Here's how the part is built. I have some questions about the finished solid (model axes, mm). Coordinates: 2 decimals unless noted, no trailing zeros. Write each loop counter-clockwise with the first axis right and the second up, starting at its lowest first coordinate (ties: lowest second). Pieces come first, ordered by that corner, then holes. Notation, with made-up numbers: (-33.75, -10.75) -> (-24.75, -10.75) arc R14 cw to (-24.75, 16.25) -> close; hole circle Ø3 at (27, 19.5). An arc over 180 degrees is marked (long way). Use a Markdown table: item, result. Add a question column.
Item 1: Imagine slicing it at C-C, the plane z = 182. Write out the boundary of the cut face in (x, y), and give its area (3 significant figures).
Item 2: If I drill on line 1 along Y through (x, z) = (0.75, 92); line 2 along X through (y, z) = (6, 53); line 3 along Y through (x, z) = (1.5, 62), over which ranges is the centre line in solid material (lowest first)? Write a range as from..to.
Item 3: Will these pins go through, and if not, where does the flat tip stop? pin 1 Ø6 at (x, y) = (-3, 0.5) entering from -Z; pin 2 Ø2 at (x, z) = (7.5, 135.5) entering from -Y; pin 3 Ø1.5 at (y, z) = (-7.5, 146) entering from +X; pin 4 Ø1.5 at (x, z) = (1, 33.5) entering from -Y.
Autodesk Inventor part; units mm, degrees
ref_plane "YZ Plane" through (0, 0, 0) normal (1, 0, 0) x (0, 1, 0)
ref_plane "XZ Plane" through (0, 0, 0) normal (0, 1, 0) x (-1, 0, 0)
ref_plane "XY Plane" through (0, 0, 0) normal (0, 0, 1) x (1, 0, 0)
sketch "Skizze1" plane through (0, 0, 0) normal (0, 0, 1) x (1, 0, 0)
  circle A0 centre (0, 0) radius 8
  circle A1 centre (0, 0) radius 10.05
  dimension "d0" = 20.1
  dimension "d1" = 2.05
extrude "Extrusion1" add sketch "Skizze1" along normal blind 286
sketch "Skizze2" plane through (0, 0, 286) normal (0, 0, 1) x (1, 0, 0)
  circle A0 centre (0, 0) radius 10.05
  circle A1 centre (0, 0) radius 9.75
  dimension "d4" = 19.5
extrude "Extrusion2" cut sketch "Skizze2" against normal through all
sketch "Skizze3" plane through (0, 0, 0) normal (0, 0, -1) x (-1, 0, 0)
  circle A0 centre (0, 0) radius 9.75
  circle A1 centre (0, 0) radius 8
  circle A2 centre (0, 0) radius 10
  dimension "d7" = 20
extrude "Extrusion3" add sketch "Skizze3" against normal blind 9 contours A2
sketch "Skizze4" plane through (0, 0, 286) normal (0, 0, 1) x (1, 0, 0)
  circle A0 centre (0, 0) radius 9.75
  circle A1 centre (0, 0) radius 8
  circle A2 centre (0, 0) radius 9
  dimension "d10" = 18
extrude "Extrusion4" cut sketch "Skizze4" against normal blind 50 contours A0
sketch "Skizze5" plane through (0, 0, 0) normal (0, 1, 0) x (-1, 0, 0)
  line L0 (-10, 9) -> (10, 9)
  line L1 (10, 0) -> (-10, 0)
  line L2 (-9.75, 236) -> (9.75, 236)
  line L3 (10, 0) -> (10, 9)
  line L4 (8, 0) -> (8, 286)
  line L5 (9.75, 236) -> (9.75, 9)
  line L6 (10, 9) -> (9.25, 9)
  line L7 (9.25, 9) -> (9.25, 7)
  line L8 (9.25, 7) -> (10, 7)
  line L9 (10, 7) -> (10, 9)
  line L10 (14, 0) -> (-14, 0)
  line L11 (0, -57.2) -> (0, 343.2)
  point P0 (0, 0)
  point P1 (9.9, 9)
  point P2 (-9.9, 9)
  point P3 (9.75, 9)
  dimension "d13" = 2
  dimension "d14" = 18.5
revolve "Umdrehung1" cut sketch "Skizze5" angle 360 about axis through (0, 0, -10) along (0, 0, 1) contours L0 L3 L8 L7
chamfer "Fase1" distance 0.75 angle 45 1 edges at (10, 0, 7)
thread "Gewinde2"
fillet "Rundung1" radius 0.5 1 edges at (-9, 0, 236)
properties part number "13_0204_024"
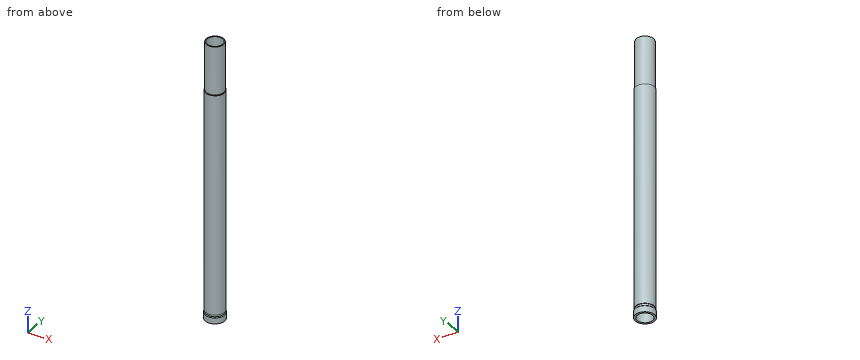
Ans:
| question | item | result |
|---|---|---|
| 1 | outline | circle Ø19.5 at (0, 0); hole circle Ø16 at (0, 0) |
| 1 | area | 97.6 mm^2 |
| 2 | line 1 | y = -9.72..-7.96, 7.96..9.72 |
| 2 | line 2 | x = -7.69..-5.29, 5.29..7.69 |
| 2 | line 3 | y = -9.63..-7.86, 7.86..9.63 |
| 3 | pin 1 | passes through |
| 3 | pin 2 | stops at y = -7.27 |
| 3 | pin 3 | stops at x = 7.04 |
| 3 | pin 4 | stops at y = -9.75 |
